Could you check a few things on this model? Use its own coordinates, in mm. A direction names the side the tool comes from. Give positions to 0.01 mm unless a question says otherwise; leave off trailing zeros. Write each loop counter-clockwise with the first axis right and the second up, starting at its lowest first coordinate (ties: lowest second). Pieces come first, ordered by that corner, then holes. Notation, with made-up numbers: M -30.5,22.5 L 17.5,22.5 A22 cw 17.5,32.5 Z; hole C -18,-13 d3. An arc over 180 degrees is marked long. Use one line per item in the form item = value.
from build123d import *

# Parameters (mm, degrees)
SHEET_EXTRUDE_1_2_DEPTH = 50
SKETCH_1_2_W            = 97.399040294
SKETCH_1_2_H            = 78.98176722
THICKEN_1_T1            = 2
SHELL_START             = -3.0000001
SHELL_1_OUTLINE_W       = 103.399040294
SHELL_1_OUTLINE_H       = 84.98176722
SHELL_1_OUTLINE_W_2     = 95.399040294
SHELL_1_OUTLINE_H_2     = 76.98176722
SHELL_1_DEPTH           = 54.0000001
SHELL_1_2_OUTLINE_W     = 95.399040294
SHELL_1_2_OUTLINE_H     = 76.98176722
SHELL_1_2_DEPTH         = 4.0000001
SHELL_START_2           = -44.324310237
SHELL_1_3_DEPTH         = 101.399040294
SHELL_1_4_OUTLINE_W     = 78.98176722
SHELL_1_4_OUTLINE_H     = 50
SHELL_1_4_DEPTH         = 2
SHELL_START_3           = 55.074730057
SHELL_1_5_OUTLINE_W     = 78.98176722
SHELL_1_5_OUTLINE_H     = 50
SHELL_1_5_DEPTH         = 2


with BuildPart() as body_1:
    # Sheet Extrude 1: a surface, the sketch's curves swept straight by 50 mm
    with BuildLine(Plane.XY, mode=Mode.PRIVATE) as sheet_extrude_1_2_path:
        Line((-42.324310237, 40.376329431), (55.074730057, 40.376329431))
        Line((55.074730057, 40.376329431), (55.074730057, -38.605437789))
        Line((55.074730057, -38.605437789), (-42.324310237, -38.605437789))
        Line((-42.324310237, -38.605437789), (-42.324310237, 40.376329431))
    sheet_extrude_1_2 = Shell.extrude(sheet_extrude_1_2_path.wire(), (0 * SHEET_EXTRUDE_1_2_DEPTH, 0 * SHEET_EXTRUDE_1_2_DEPTH, 1 * SHEET_EXTRUDE_1_2_DEPTH))
    # Эскиз1<2> → Sheet Fill 1: a flat surface bounded by the sketch
    with BuildSketch(Plane.XY, mode=Mode.PRIVATE) as sheet_fill_1_3_region:
        with Locations((6.37520991, 0.885445821)):
            Rectangle(SKETCH_1_2_W, SKETCH_1_2_H)
    sheet_fill_1_3 = sheet_fill_1_3_region.sketch.faces()[0]
    # Knit 1: the surfaces knitted into one
    knit_1_1 = Shell(Face.sew_faces(sheet_extrude_1_2.faces() + sheet_fill_1_3.faces())[0])
    add(Solid.thicken(knit_1_1, THICKEN_1_T1))

    # Оболочка1: read off the stored shape, not the designer's step
    # Оболочка1 outline → Оболочка1 (add)
    with BuildSketch(Plane.XY.offset(SHELL_START)):
        with Locations((6.37520991, 0.885445821)):
            Rectangle(SHELL_1_OUTLINE_W, SHELL_1_OUTLINE_H)
        with Locations((6.37520991, 0.885445821)):
            Rectangle(SHELL_1_OUTLINE_W_2, SHELL_1_OUTLINE_H_2, mode=Mode.SUBTRACT)
    extrude(amount=SHELL_1_DEPTH)

    # Shell 1 2 outline → Shell 1 2 (add)
    with BuildSketch(Plane.XY.offset(SHELL_START)):
        with Locations((6.37520991, 0.885445821)):
            Rectangle(SHELL_1_2_OUTLINE_W, SHELL_1_2_OUTLINE_H)
    extrude(amount=SHELL_1_2_DEPTH)

    # Shell 1 3 outline → Shell 1 3 (cut)
    with BuildSketch(Plane.YZ.offset(SHELL_START_2)):
        with BuildLine():
            add(Edge.make_bspline(
                [(42.376329431, -2), (-40.605437789, -2)],
                knots=[-0.0253223, -0.0253223, 1.0253223, 1.0253223], degree=1))
            Line((42.376329431, -2), (42.376329431, 50))
            Line((42.376329431, 50), (40.376329431, 50))
            Line((40.376329431, 50), (40.376329431, 0))
            Line((40.376329431, 0), (-38.605437789, 0))
            Line((-38.605437789, 0), (-38.605437789, 50))
            Line((-38.605437789, 50), (-40.605437789, 50))
            Line((-40.605437789, 50), (-40.605437789, -2))
        make_face()
    extrude(amount=SHELL_1_3_DEPTH, mode=Mode.SUBTRACT)

    # Shell 1 4 outline → Shell 1 4 (cut)
    with BuildSketch(Plane.YZ.offset(SHELL_START_2)):
        with Locations((0.885445821, 25)):
            Rectangle(SHELL_1_4_OUTLINE_W, SHELL_1_4_OUTLINE_H)
    extrude(amount=SHELL_1_4_DEPTH, mode=Mode.SUBTRACT)

    # Shell 1 5 outline → Shell 1 5 (cut)
    with BuildSketch(Plane.YZ.offset(SHELL_START_3)):
        with Locations((0.885445821, 25)):
            Rectangle(SHELL_1_5_OUTLINE_W, SHELL_1_5_OUTLINE_H)
    extrude(amount=SHELL_1_5_DEPTH, mode=Mode.SUBTRACT)


solid = body_1.part
1) If I drill on L1, parallel to Y at x = -9, z = 22; L2, parallel to X at y = 13, z = 26.5; L3, parallel to Y at x = -7, z = 0.5, over which ranges is the centre line in solid material (lowest first)?
Checked values:
L1 = -41.61 to -40.61, -38.61 to -37.61, 39.38 to 40.38, 42.38 to 43.38
L2 = -45.32 to -44.32, -42.32 to -41.32, 54.07 to 55.07, 57.07 to 58.07
L3 = -41.61 to -40.61, -38.61 to 40.38, 42.38 to 43.38
2) For faces 4 (the flat face through (6, 1, -3)), 5 (the flat face through (6, 39.376, 26)), 6 (the flat face through (6, -40.605, 24)), which set-ups out of +Z, -Z, +X, -X, +Y, -Y let a thin tool reach every point of the face, with its end or its side?
Checked values:
face_4 = -Z, +X, -X, +Y, -Y
face_5 = +Z
face_6 = none
3) I want a section at A-A, the plane z = 47.5. Please give me the cut outline in (x, y).
Checked values:
outline = M -45.32,-41.61 L 58.07,-41.61 L 58.07,43.38 L -45.32,43.38 Z; M -42.32,-38.61 L 55.07,-38.61 L 55.07,40.38 L -42.32,40.38 Z; hole M -44.32,-40.61 L 57.07,-40.61 L 57.07,42.38 L -44.32,42.38 Z; hole M -41.32,-37.61 L 54.07,-37.61 L 54.07,39.38 L -41.32,39.38 Z
4) Thinking about a two-plate mould opening in Y: for faces 1 (the flat face through (2, -40, 51)), 2 (the flat face through (6, 42.376, 24)), 3 (the flat face through (6, -41.605, 24)), which applies, released by +Y, released by -Y, zero draft, split by the parting line, or undercut?
Checked values:
face_1 = zero draft
face_2 = undercut
face_3 = released by -Y
5) For pin 1 Ø4 at (x, y) = (10.5, -17.5) entering from +Z, with a flat end and sliding along its axis, tell me the tip position at first contact or that it passes through.
Checked values:
pin_1 = 1
